The listing builds one solid part. Answer for the finished solid, in the listing's coordinates (mm). Coordinates: 2 decimals unless noted, no trailing zeros. Order: outer loops, then holes, each group sorted by start corner. A loop starts at its lowest first (then second) coordinate and runs counter-clockwise, first axis right, second up. Notation, with made-up numbers: (-40, 30.5) - (0, 30.5) arc R28 cw to (0, 67.5) - close; hole circle Ø5 at (56.5, -37). An arc over 180 degrees is marked (long way). One line per item, written item: value. Start each with the question number.
```python
from build123d import *

# Parameters (mm, degrees)
SKETCH1_W           = 1070
SKETCH1_H           = 350
BOSS_EXTRUDE1_DEPTH = 6
SKETCH2_R           = 2.5
CUT_EXTRUDE1_DEPTH  = 618.483603021


with BuildPart() as part:
    # Sketch1 → Boss-Extrude1 (new body)
    with BuildSketch(Plane.XY):
        Polygon((575, -215), (575, 175), (575, 225), (535, 225), (-535, 225), (-575, 225), (-575, 175), (-575, -215), align=None)
        Rectangle(SKETCH1_W, SKETCH1_H, mode=Mode.SUBTRACT)
    extrude(amount=BOSS_EXTRUDE1_DEPTH)

    # Sketch2 → Cut-Extrude1 (cut, through all)
    with BuildSketch(Plane.XY.offset(6)):
        with Locations((-555, 210)):
            Circle(SKETCH2_R)
        with Locations((-555, -205)):
            Circle(SKETCH2_R)
        with Locations((555, -205)):
            Circle(SKETCH2_R)
        with Locations((555, 210)):
            Circle(SKETCH2_R)
    extrude(amount=-CUT_EXTRUDE1_DEPTH, mode=Mode.SUBTRACT)


solid = part.part
```
(1) The part is cut by section C-C on x = 343. Determine the outline of the cut face in (y, z).
(2) The part is cut by section A-A on z = 1.15. Determine the outline of the cut face in (x, y), plus the area to 3 significant figures.
(3) The part is cut by section B-B on y = 39.5. Determine the outline of the cut face in (x, z).
(4) Consider probe 1 along Y at (x, z) = (555, 2.85); probe 2 along X at (y, z) = (210, 1.3); probe 3 along Y at (x, z) = (-506, 0.95). Determine where each line is inside the solid, lowest interval first.
Completed:
1. outline: (-215, 0) - (-175, 0) - (-175, 6) - (-215, 6) - close; (175, 0) - (225, 0) - (225, 6) - (175, 6) - close
2. outline: (-575, -215) - (575, -215) - (575, 225) - (-575, 225) - close; hole circle Ø5 at (-555, -205); hole circle Ø5 at (-555, 210); hole (-535, -175) - (535, -175) - (535, 175) - (-535, 175) - close; hole circle Ø5 at (555, -205); hole circle Ø5 at (555, 210)
2. area: 131,000 mm2
3. outline: (-575, 0) - (-535, 0) - (-535, 6) - (-575, 6) - close; (535, 0) - (575, 0) - (575, 6) - (535, 6) - close
4. probe 1: y = -215 to -207.5, -202.5 to 207.5, 212.5 to 225
4. probe 2: x = -575 to -557.5, -552.5 to 552.5, 557.5 to 575
4. probe 3: y = -215 to -175, 175 to 225
